Verification items for the finished model (mm, model axes). Face numbers are marked on the shaded views. A direction names the side the tool comes from. Give positions to 0.01 mm unless a question says otherwise; leave off trailing zeros. Order: outer loops, then holes, each group sorted by start corner. A loop starts at its lowest first (then second) coordinate and runs counter-clockwise, first axis right, second up. Notation, with made-up numbers: (-11.75, -32) -> (35.25, -32) arc R7 cw to (35.25, -22) -> close; hole circle Ø7 at (72.5, 82). An arc over 180 degrees is marked (long way). Return JSON: item names as keys, results as strings. Group by question number.
(1) Release check for a two-part mould opening along X. For the marked faces 1, 2 and 3 record: pulls with the +X half, pulls with the -X half, needs draft (parallel to the pull), parting line crosses it, or undercut.
(2) Thickness scan on line 1 along Z through (x, y) = (-26, 0); line 2 along Z through (x, y) = (28.5, 18.5); line 3 along Z through (x, y) = (-44.5, -1.5). Record the ranges inside material, lowest first.
(3) Cross-section at B-B on y = 0. Enter the section's corners in (x, z), then the cut area to 3 significant figures.
(4) Cross-section at D-D on x = -120. Enter the section's corners in (y, z).
(5) Cross-section at A-A on z = -18.5. Enter the section's corners in (x, y).
(6) Tool access check on the marked faces 4, 5 and 6. Record the directions out of +Z, -Z, +X, -X, +Y, -Y that give a thin tool (end or side, any length) a straight path to the whole face; none if there is none.
(7) Depth check by flat-ended pin: pin 1 Ø9 at (x, y) = (-70.5, -0.5) entering from -Z; pin 2 Ø12 at (y, z) = (17, -35) entering from +X. Enter the tip coordinate at first touch or a pass-through.
(8) Cross-section at C-C on x = -95.5. Enter the section's corners in (y, z).
from build123d import *

# Parameters (mm, degrees)
BOSS_EXTRUDE1_DEPTH = 38.1
CUT_EXTRUDE1_START  = -5.08
CUT_EXTRUDE1_DEPTH  = 5.08
SWEEP1_START        = -8.89
SWEEP1_DEPTH        = 17.78


# Read off the part's stored shape, not the designer's step: Sweep1
with BuildPart() as part:
    # Sketch2 → Revolve1 (revolve)
    with BuildSketch(Plane(origin=(0, 0, 0), x_dir=(1, 0, 0), z_dir=(0, 1, 0))):
        Polygon((0, 50.8), (38.1, 50.8), (34.433825791, 44.45), (19.193825791, 44.45), (15.527651581, 38.1), (0, 38.1), align=None)
    revolve(axis=Axis((0, 0, 0), (0, 0, -1)))

    # Sketch3 → Boss-Extrude1 (add)
    with BuildSketch(Plane.XY.offset(-38.1)):
        with BuildLine():
            Line((0, 8.89), (-10.640962008, 3.383819151))
            ThreePointArc((-10.640962008, 3.383819151), (-12.7, 0), (-10.640962008, -3.383819151))
            Line((-10.640962008, -3.383819151), (0, -8.89))
            ThreePointArc((0, -8.89), (8.89, 0), (0, 8.89))
        make_face()
    extrude(amount=BOSS_EXTRUDE1_DEPTH)

    # Sketch4 → Cut-Extrude1 (cut)
    with BuildSketch(Plane.XY.offset(CUT_EXTRUDE1_START)):
        with BuildLine():
            Line((0, 8.89), (0, -8.89))
            Line((0, -8.89), (-10.640962008, -3.383819151))
            ThreePointArc((-10.640962008, -3.383819151), (-12.7, 0), (-10.640962008, 3.383819151))
            Line((-10.640962008, 3.383819151), (0, 8.89))
        make_face()
    extrude(amount=CUT_EXTRUDE1_DEPTH, mode=Mode.SUBTRACT)

    # Sweep1 outline → Sweep1 (add)
    with BuildSketch(Plane(origin=(0, 0, 0), x_dir=(1, 0, 0), z_dir=(0, 1, 0)).offset(SWEEP1_START)):
        with BuildLine():
            Line((-103.886, 0), (0, 0))
            Line((0, 0), (0, 5.08))
            Line((0, 5.08), (-103.886, 5.08))
            ThreePointArc((-103.886, 5.08), (-111.662127346, 6.626767899), (-118.254409794, 11.031590206))
            Line((-118.254409794, 11.031590206), (-142.321496198, 35.098676611))
            Line((-142.321496198, 35.098676611), (-145.913598647, 31.506574162))
            Line((-145.913598647, 31.506574162), (-121.846512242, 7.439487758))
            ThreePointArc((-121.846512242, 7.439487758), (-113.606159182, 1.933459874), (-103.886, 0))
        make_face()
    extrude(amount=SWEEP1_DEPTH)


solid = part.part
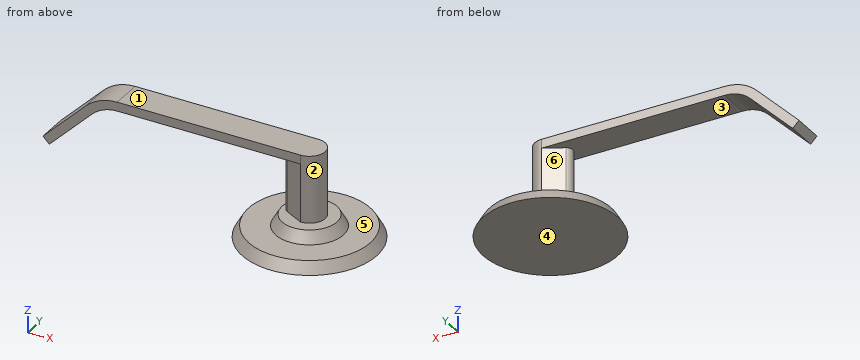
Verdict:
{
 "1": {"face 1": "needs draft", "face 2": "pulls with the +X half", "face 3": "undercut"},
 "2": {"line 1": "-50.8 to -44.45, -5.08 to 0", "line 2": "-50.8 to -44.45", "line 3": "-5.08 to 0"},
 "3": {"outline": "(-145.91, -31.51) -> (-142.32, -35.1) -> (-118.25, -11.03) arc R20.32 cw to (-103.89, -5.08) -> (-12.7, -5.08) -> (-12.7, -38.1) -> (-15.53, -38.1) -> (-19.19, -44.45) -> (-34.43, -44.45) -> (-38.1, -50.8) -> (38.1, -50.8) -> (34.43, -44.45) -> (19.19, -44.45) -> (15.53, -38.1) -> (8.89, -38.1) -> (8.89, 0) -> (-103.89, 0) arc R25.4 ccw to (-121.85, -7.44) -> close", "area": "2,230 mm²"},
 "4": {"outline": "(-8.89, -12.78) -> (8.89, -12.78) -> (8.89, -5.77) -> (-8.89, -5.77) -> close"},
 "5": {"outline": "(-132.91, -8.89) -> (-125.72, -8.89) -> (-125.72, 8.89) -> (-132.91, 8.89) -> close; (-10.64, -3.38) -> (0, -8.89) arc R8.89 ccw to (0, 8.89) -> (-10.64, 3.38) arc R3.81 ccw to start"},
 "6": {"face 4": "-Z, +X, -X, +Y, -Y", "face 5": "none", "face 6": "+Y"},
 "7": {"pin 1": "z = -5.08", "pin 2": "x = 10.07"},
 "8": {"outline": "(-8.89, -5.08) -> (8.89, -5.08) -> (8.89, 0) -> (-8.89, 0) -> close"}
}
